from build123d import *

# Parameters (mm, degrees)
SKETCH1_R           = 5.5
BOSS_EXTRUDE1_DEPTH = 5
CUT_EXTRUDE3_DEPTH  = 5


with BuildPart() as part:
    # Sketch1 → Boss-Extrude1 (new body)
    with BuildSketch(Plane.XY):
        Circle(SKETCH1_R)
    extrude(amount=BOSS_EXTRUDE1_DEPTH)

    # Sketch2 → Cut-Extrude3 (cut)
    with BuildSketch(Plane.XY.offset(5)):
        with BuildLine():
            Line((0, 0), (-1.972639316, 0.329687929))
            Line((-1.972639316, 0.329687929), (-2.817213309, -4.723696558))
            add(Edge.make_bspline(
                [(-2.817213309, -4.723696558), (-2.331717092, -5.013604459), (-1.497847825, -5.349651617), (-0.517167494, -5.488823483), (0.280656275, -5.510097286), (0.757829967, -5.460753651), (1.128065322, -5.383072415)],
                knots=[0, 0, 0, 0, 0.414681005, 0.650712608, 0.722388742, 1, 1, 1, 1], degree=3))
            Line((1.128065322, -5.383072415), (1.972639316, -0.329687929))
            Line((1.972639316, -0.329687929), (0, 0))
        make_face()
    extrude(amount=-CUT_EXTRUDE3_DEPTH, mode=Mode.SUBTRACT)


with BuildPart() as cut_extrude3_kept_piece:
    # of the separate pieces the step leaves, the one the design keeps (cut_extrude3_pieces_kept)
    add(part.part.solids().sort_by_distance((1.128065322, -5.383072415, 0))[0])


solid = cut_extrude3_kept_piece.part
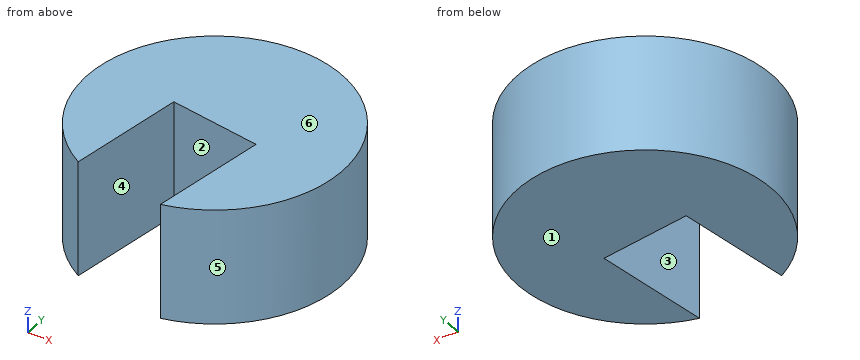
CAD build for the part. Positions are in the model's coordinates, mm. Face numbers are marked on the shaded views. A direction names the side the tool comes from. Round coordinates to 2 decimals unless told otherwise and drop trailing zeros. Write each loop counter-clockwise with the first axis right and the second up, starting at its lowest first coordinate (ties: lowest second). Pieces come first, ordered by that corner, then holes.
(1) Slice it at C-C, the plane z = 2.5. Write the cut outline in (x, y), and give its area (3 significant figures).
(2) 3-axis set-ups, long thin cutter, end or side, ignore diameter. For the marked faces 1 and 2: which of +Z, -Z, +X, -X, +Y, -Y reach the whole face in a straight line?
(3) Slice it at B-B, the plane x = 1.75. Write the cut outline in (y, z).
(4) Drop flat-ended pins along their axis: P1, Ø2, axis at y = 3.5, z = 1, coming from the -X side; P2, Ø2, axis at x = 4, z = 2, coming from the -Y side; P3, Ø1.5, axis at x = -4, z = 4.5, coming from the -Y side. Give the stop position or say it passes through.
(5) Probe line 1 along Y through (x, z) = (-3.5, 3.25); line 2 along Y through (x, z) = (-4, 2.9); line 3 along X through (y, z) = (-4.5, 1.3). List the from-to ranges inside material, lowest first.
(6) Mould opens along Y. For the marked faces 3, 4, 5 and 6 say: pulls with the +Y half, pulls with the -Y half, needs draft (parallel to the pull), parting line crosses it, or undercut.
(7) Slice it at D-D, the plane x = 0. Write the cut outline in (y, z), and give its area (3 significant figures).
(8) Slice it at A-A, the plane y = -1.25. Write the cut outline in (x, z), and give its area (3 significant figures).
From the geometry:
1. outline: (-2.82, -4.72) - (-1.97, 0.33) - (1.97, -0.33) - (1.13, -5.38) arc R5.5 ccw (long way) to start
1. area: 73.5 mm2
2. face 1: -Z, +X, -X, +Y, -Y
2. face 2: +Z, -Z
3. outline: (-5.21, 0) - (-1.66, 0) - (-1.66, 5) - (-5.21, 5) - close; (-0.29, 0) - (5.21, 0) - (5.21, 5) - (-0.29, 5) - close
4. P1: stops at x = -4.9
4. P2: stops at y = -4.61
4. P3: stops at y = -4.44
5. line 1: y = -4.24 to 4.24
5. line 2: y = -3.77 to 3.77
5. line 3: x = -3.16 to -2.78, 1.28 to 3.16
6. face 3: undercut
6. face 4: pulls with the -Y half
6. face 5: parting line crosses it
6. face 6: needs draft
7. outline: (0, 0) - (5.5, 0) - (5.5, 5) - (0, 5) - close
7. area: 27.5 mm2
8. outline: (-5.36, 0) - (-2.24, 0) - (-2.24, 5) - (-5.36, 5) - close; (1.82, 0) - (5.36, 0) - (5.36, 5) - (1.82, 5) - close
8. area: 33.3 mm2
